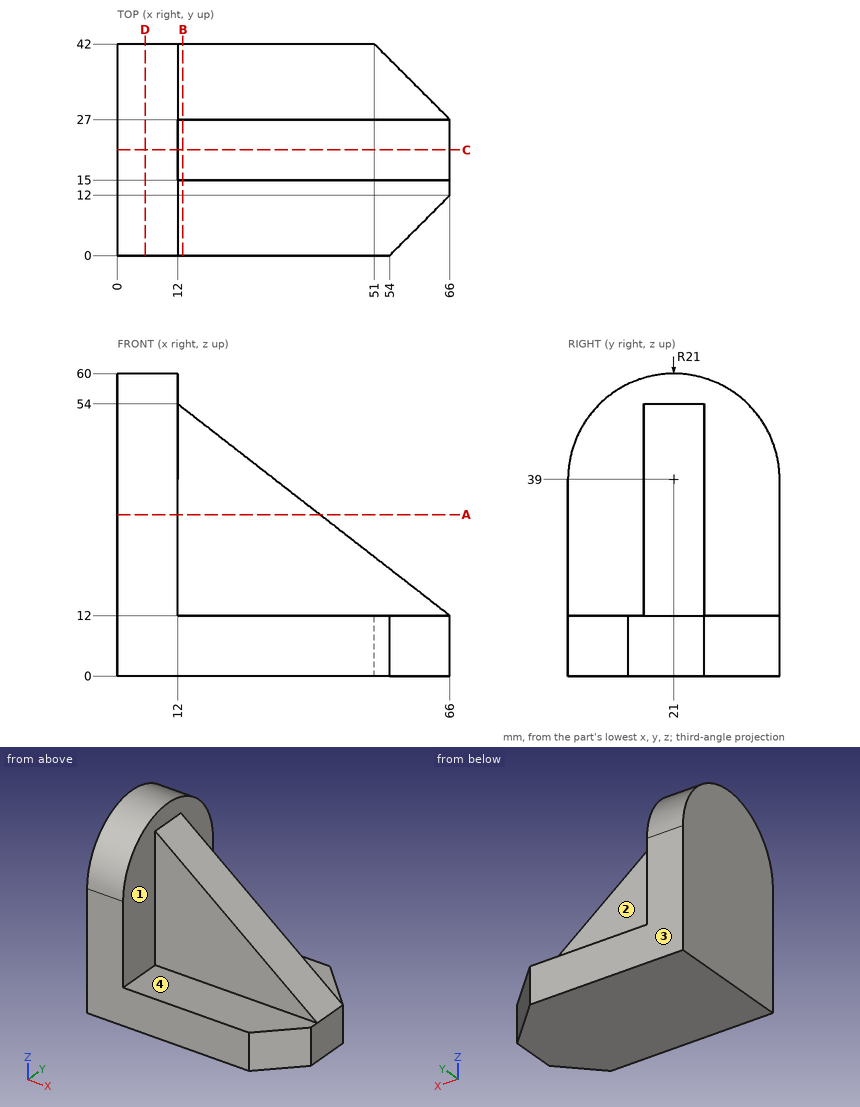
Job drawing, mm, ordinate dimensions from the low corner. One solid piece. A direction names the side the tool comes from. Round coordinates to 2 decimals unless told otherwise and drop trailing zeros. Write each loop counter-clockwise with the first axis right and the second up, starting at its lowest first coordinate (ties: lowest second). Pieces come first, ordered by that corner, then holes. Notation, with made-up numbers: M 67,-29 L 100,-29 A11 ccw 100,-17 Z; hole C 50.25,8 d6. An arc over 180 degrees is marked long. Return JSON: item names as keys, results as strings. Group by question number.
(1) Saw through at A-A on z = 32. Write the cut outline in (x, y), then the cut area to 3 significant figures.
(2) Pin check, flat tips, straight feed: pin 1 Ø12 at (x, y) = (48, 36) entering from +Z; pin 2 Ø3 at (y, z) = (35, 45.5) entering from +X; pin 3 Ø10 at (y, z) = (11.5, 20) entering from +X. Stop position of each tip, or through.
(3) Drill centre lines: probe 1 along Y at (x, z) = (56, 18.5); probe 2 along X at (y, z) = (7, 25.5). Where is each one in solid material? Low to high.
(4) Saw through at C-C on y = 21. Write the cut outline in (x, z).
(5) Which spindle directions (+Z, -Z, +X, -X, +Y, -Y) get a long thin tool onto all of the face, cutting with end or side? Do the marked faces 1, 2, 3 and 4. Say none if no direction does.
(6) Saw through at D-D on x = 5.5. Write the cut outline in (y, z).
(7) Saw through at B-B on x = 13. Write the cut outline in (y, z).
Returned:
{
 "1": {"outline": "M 0,0 L 12,0 L 12,15 L 40.29,15 L 40.29,27 L 12,27 L 12,42 L 0,42 Z", "area": "843 mm²"},
 "2": {"pin 1": "z = 12", "pin 2": "x = 12", "pin 3": "x = 60.31"},
 "3": {"probe 1": "15 to 27", "probe 2": "0 to 12"},
 "4": {"outline": "M 0,0 L 66,0 L 66,12 L 12,54 L 12,60 L 0,60 Z"},
 "5": {"face 1": "+Z, +X", "face 2": "+Z, +X, +Y", "face 3": "+Z, -Z, +X, -X, +Y", "face 4": "+Z, +X, -Y"},
 "6": {"outline": "M 0,0 L 42,0 L 42,39 A21 ccw 0,39 Z"},
 "7": {"outline": "M 0,0 L 42,0 L 42,12 L 27,12 L 27,53.22 L 15,53.22 L 15,12 L 0,12 Z"}
}
